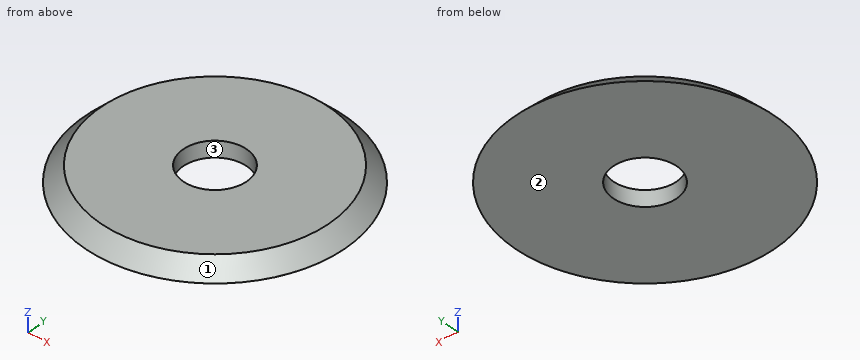
Autodesk Inventor part; units mm, degrees
ref_plane "YZ Plane" through (0, 0, 0) normal (1, 0, 0) x (0, 1, 0)
ref_plane "XZ Plane" through (0, 0, 0) normal (0, 1, 0) x (-1, 0, 0)
ref_plane "XY Plane" through (0, 0, 0) normal (0, 0, 1) x (1, 0, 0)
sketch "スケッチ1" plane through (0, 0, 0) normal (0, 0, 1) x (1, 0, 0)
  circle A0 centre (0, 0) radius 4.1
  dimension "d0" = 8.2
extrude "押し出し1" add sketch "スケッチ1" along normal blind 1
chamfer "面取り1" distance 1 angle 45 1 edges at (-4.1, 0, 1) measured on face at (0.2975, 0.2635, 1)
sketch "スケッチ2" plane through (0, 0, 1) normal (0, 0, 1) x (1, 0, 0)
  circle A0 centre (0, 0) radius 1
  dimension "d6" = 2
extrude "押し出し2" cut sketch "スケッチ2" against normal blind 1
sketch "スケッチ3" plane through (0, 0, 1) normal (0, 0, 1) x (1, 0, 0)
  circle A0 centre (0, 0) radius 4.8361
extrude "押し出し3" cut sketch "スケッチ3" against normal blind 0.5
properties part number "blade" material "ステンレス鋼"
Could you check a few things on this model? Use its own coordinates, in mm. Face numbers are marked on the shaded views. Give positions to 0.01 mm unless a question says otherwise; leave off trailing zeros. Order: outer loops, then holes, each group sorted by start corner. A loop starts at its lowest first (then second) coordinate and runs counter-clockwise, first axis right, second up. Notation, with made-up numbers: (62, 77.5) -> (83, 77.5) arc R30 ccw to (83, 112.5) -> close; hole circle Ø9 at (84.25, -40). An arc over 180 degrees is marked (long way). Answer in a Markdown table with one row per item. Add a question column.
Item 1: Please list where these lines run through material, in increasing order: probe 1 along X at (y, z) = (0.5, 0.4); probe 2 along Y at (x, z) = (-2.25, 0.35); probe 3 along X at (y, z) = (1.5, 0.15).
Item 2: Imagine slicing it at C-C (z = 0.3). List the corners of the cut face in (x, y) for me, and give its area (3 significant figures).
Item 3: We'd pull the mould along Y, two halves only. Please class the marked faces 1, 2 and 3: pulls with the +Y half, pulls with the -Y half, needs draft (parallel to the pull), parting line crosses it, or undercut.
Result:
| question | item | result |
|---|---|---|
| 1 | probe 1 | -3.67 to -0.87, 0.87 to 3.67 |
| 1 | probe 2 | -3 to 3 |
| 1 | probe 3 | -3.65 to 3.65 |
| 2 | outline | circle Ø7.6 at (0, 0); hole circle Ø2 at (0, 0) |
| 2 | area | 42.2 mm2 |
| 3 | face 1 | parting line crosses it |
| 3 | face 2 | needs draft |
| 3 | face 3 | undercut |
